Could you check a few things on this model? Use its own coordinates, in mm. A direction names the side the tool comes from. Give positions to 0.01 mm unless a question says otherwise; leave off trailing zeros. Order: outer loops, then holes, each group sorted by start corner. A loop starts at its lowest first (then second) coordinate and runs counter-clockwise, first axis right, second up.
from build123d import *

# Parameters (mm, degrees)
SKETCH1_R           = 7
SKETCH1_R_2         = 5
SKETCH1_R_3         = 1.5
SKETCH1_R_4         = 2.75
SKETCH1_R_5         = 1.65
BOSS_EXTRUDE1_DEPTH = 5


with BuildPart() as part:
    # Sketch1 → Boss-Extrude1 (new body)
    with BuildSketch(Plane.XY):
        with BuildLine():
            Line((61, -35), (-61, -35))
            ThreePointArc((-61, -35), (-96, 0), (-61, 35))
            Line((-61, 35), (61, 35))
            ThreePointArc((61, 35), (96, 0), (61, -35))
        make_face()
        with Locations((61, 0)):
            Circle(SKETCH1_R, mode=Mode.SUBTRACT)
        with Locations((-61, 0)):
            Circle(SKETCH1_R_2, mode=Mode.SUBTRACT)
        with Locations((-61, -29)):
            Circle(SKETCH1_R_3, mode=Mode.SUBTRACT)
        with Locations((-61, 29)):
            Circle(SKETCH1_R_3, mode=Mode.SUBTRACT)
        with Locations((61, 29)):
            Circle(SKETCH1_R_3, mode=Mode.SUBTRACT)
        with Locations((61, -29)):
            Circle(SKETCH1_R_3, mode=Mode.SUBTRACT)
        with Locations((0, -29)):
            Circle(SKETCH1_R_3, mode=Mode.SUBTRACT)
        with Locations((0, 29)):
            Circle(SKETCH1_R_3, mode=Mode.SUBTRACT)
        with Locations((-61, 18.25)):
            Circle(SKETCH1_R_4, mode=Mode.SUBTRACT)
        with Locations((-61, -18.25)):
            Circle(SKETCH1_R_4, mode=Mode.SUBTRACT)
        with Locations((-90, 0)):
            Circle(SKETCH1_R_3, mode=Mode.SUBTRACT)
        with Locations((-32, 0)):
            Circle(SKETCH1_R_3, mode=Mode.SUBTRACT)
        with Locations((90, 0)):
            Circle(SKETCH1_R_3, mode=Mode.SUBTRACT)
        with Locations((32, 0)):
            Circle(SKETCH1_R_3, mode=Mode.SUBTRACT)
        with Locations((68, -15.5)):
            Circle(SKETCH1_R_3, mode=Mode.SUBTRACT)
        with Locations((68, 15.5)):
            Circle(SKETCH1_R_5, mode=Mode.SUBTRACT)
        with Locations((54.630491741, 7.75587519)):
            Circle(SKETCH1_R_5, mode=Mode.SUBTRACT)
        with Locations((54.630491741, -7.75587519)):
            Circle(SKETCH1_R_5, mode=Mode.SUBTRACT)
        with Locations((81.369508259, -7.75587519)):
            Circle(SKETCH1_R_5, mode=Mode.SUBTRACT)
        with Locations((81.369508259, 7.75587519)):
            Circle(SKETCH1_R_5, mode=Mode.SUBTRACT)
        with BuildLine():
            Line((2.25, -6.25), (2.25, -16.25))
            ThreePointArc((2.25, -16.25), (0, -18.5), (-2.25, -16.25))
            Line((-2.25, -16.25), (-2.25, -6.25))
            ThreePointArc((-2.25, -6.25), (0, -4), (2.25, -6.25))
        make_face(mode=Mode.SUBTRACT)
        with BuildLine():
            Line((-24.76, 10), (-9.76, 10))
            ThreePointArc((-9.76, 10), (-7.26, 7.5), (-9.76, 5))
            Line((-9.76, 5), (-24.76, 5))
            ThreePointArc((-24.76, 5), (-27.26, 7.5), (-24.76, 10))
        make_face(mode=Mode.SUBTRACT)
        with BuildLine():
            Line((-24.76, 20.24), (-9.76, 20.24))
            ThreePointArc((-9.76, 20.24), (-7.26, 17.74), (-9.76, 15.24))
            Line((-9.76, 15.24), (-24.76, 15.24))
            ThreePointArc((-24.76, 15.24), (-27.26, 17.74), (-24.76, 20.24))
        make_face(mode=Mode.SUBTRACT)
        with BuildLine():
            Line((14.09, 10), (29.09, 10))
            ThreePointArc((29.09, 10), (31.59, 7.5), (29.09, 5))
            Line((29.09, 5), (14.09, 5))
            ThreePointArc((14.09, 5), (11.59, 7.5), (14.09, 10))
        make_face(mode=Mode.SUBTRACT)
        with BuildLine():
            Line((14.09, 20.24), (29.09, 20.24))
            ThreePointArc((29.09, 20.24), (31.59, 17.74), (29.09, 15.24))
            Line((29.09, 15.24), (14.09, 15.24))
            ThreePointArc((14.09, 15.24), (11.59, 17.74), (14.09, 20.24))
        make_face(mode=Mode.SUBTRACT)
    extrude(amount=BOSS_EXTRUDE1_DEPTH)


solid = part.part
Item 1: We'd pull the mould along Y, two halves only. Please class faces 3 (the cylindrical face through (56.155, -8.388, 2.465)), 4 (the flat face through (1, 0, 0)), 5 (the cylindrical face through (95.99, 0.77, 2.46)): +Y half, -Y half, draft (parallel to the pull), parting line (faces both ways), or undercut.
Findings:
face 3: undercut
face 4: draft
face 5: parting line
Item 2: Imagine slicing it at B-B on z = 2.8. Give the number of separate pieces and of enclosed holes in the cut face, then the cut area to 3 significant figures.
Findings:
separate pieces: 1
enclosed holes: 25
area: 11,500 mm2
Item 3: Please list where these lines run through material, in increasing order: line 1 along Y through (x, z) = (-20, 0.4); line 2 along Y through (x, z) = (61, 3.3); line 3 along X through (y, z) = (4, 3.25).
Findings:
line 1: y = -35 to 5, 10 to 15.24, 20.24 to 35
line 2: y = -35 to -30.5, -27.5 to -7, 7 to 27.5, 30.5 to 35
line 3: x = -95.77 to -64, -58 to 55.26, 66.74 to 95.77
Item 4: Imagine slicing it at A-A on x = -14.5. List the corners of the cut face in (y, z) for me.
Findings:
outline: (-35, 0) - (5, 0) - (5, 5) - (-35, 5) - close; (10, 0) - (15.24, 0) - (15.24, 5) - (10, 5) - close; (20.24, 0) - (35, 0) - (35, 5) - (20.24, 5) - close
Item 5: For faces 1 (the cylindrical face through (31.59, 7.55, 2.46)), 2 (the flat face through (1, 0, 5)), which set-ups out of +Z, -Z, +X, -X, +Y, -Y let a thin tool reach every point of the face, with its end or its side?
Findings:
face 1: +Z, -Z
face 2: +Z, +X, -X, +Y, -Y
Item 6: For pin 1 (1.5 mm diameter, centred on y = -12.5, z = 1.5, fed in from -X), with a flat end and sliding along its axis, tell me the tip position at first contact or that it passes through.
Findings:
pin 1: stops at x = -93.97
